Work out the finished part from the listing and answer in its coordinate system (mm). Round coordinates to 2 decimals unless told otherwise and drop trailing zeros. Write each loop counter-clockwise with the first axis right and the second up, starting at its lowest first coordinate (ties: lowest second). Pieces come first, ordered by that corner, then holes. Notation, with made-up numbers: (46.5, 1.25) - (52.5, 1.25) arc R27 ccw to (52.5, 28.25) - close; hole circle Ø1 at (17, -40). An arc over 180 degrees is marked (long way). Write item = value, one per line. Start each with the question number.
from build123d import *

# Parameters (mm, degrees)
SKETCH2_R                    = 12.7
BOSS_EXTRUDE1_DEPTH          = 0.79375
SKETCH3_R                    = 9.525
CUT_EXTRUDE1_DEPTH           = 1.79375
SKETCH4_W                    = 22.318168974
SKETCH4_H                    = 8.357131245
CUT_REVOLVE1_ANGLE           = 45
CUT_REVOLVE1_OTHER_WAY_ANGLE = 45


with BuildPart() as part:
    # Sketch2 → Boss-Extrude1 (new body)
    with BuildSketch(Plane(origin=(0, 0, 0), x_dir=(1, 0, 0), z_dir=(0, 1, 0))):
        Circle(SKETCH2_R)
    extrude(amount=BOSS_EXTRUDE1_DEPTH)

    # Sketch3 → Cut-Extrude1 (cut, through all)
    with BuildSketch(Plane(origin=(0, 0.79375, 0), x_dir=(1, 0, 0), z_dir=(0, 1, 0))):
        Circle(SKETCH3_R)
    extrude(amount=-CUT_EXTRUDE1_DEPTH, mode=Mode.SUBTRACT)

    # Sketch4 → Cut-Revolve1 (revolve, cut)
    with BuildSketch(Plane(origin=(0, 0, 0), x_dir=(0, 0, -1), z_dir=(1, 0, 0))):
        with Locations((-11.159084487, 3.258563731)):
            Rectangle(SKETCH4_W, SKETCH4_H)
    revolve(axis=Axis((0, -0.920001892, 0), (0, 1, 0)), revolution_arc=CUT_REVOLVE1_ANGLE, mode=Mode.SUBTRACT)

    # Sketch4 → Cut-Revolve1 other way (revolve, cut)
    with BuildSketch(Plane(origin=(0, 0, 0), x_dir=(0, 0, -1), z_dir=(1, 0, 0))):
        with Locations((-11.159084487, 3.258563731)):
            Rectangle(SKETCH4_W, SKETCH4_H)
    revolve(axis=Axis((0, -0.920001892, 0), (0, -1, 0)), revolution_arc=CUT_REVOLVE1_OTHER_WAY_ANGLE, mode=Mode.SUBTRACT)


solid = part.part
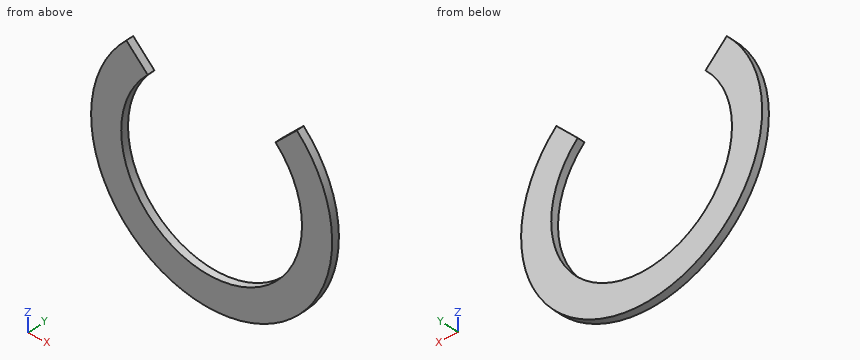
1. Consider line 1 (X direction, y = 0.5, z = 0) (3 decimals); line 2 (Z direction, x = 0, y = 0.55) (3 decimals); line 3 (Z direction, x = 8.5, y = 0.6). Determine where each line is inside the solid, lowest interval first.
2. Find section B-B on x = 7.25. Give the vertices of the cut face in (y, z).
3. Find section A-A on z = 0. Give the vertices of the cut face in (x, y) (3 decimals).
4. Find section C-C on y = 0.15. Give the vertices of the cut face in (x, z) (3 decimals).
5. Find section D-D on x = 0. Give the vertices of the cut face in (y, z) (3 decimals).
Answer key:
q1.line_1 = -12.7 to -9.525, 9.525 to 12.7
q1.line_2 = -12.7 to -9.525
q1.line_3 = -9.44 to -4.3, 4.3 to 8.5
q2.outline = (0, -10.43) - (0.79, -10.43) - (0.79, -6.18) - (0, -6.18) - close; (0, 6.18) - (0.79, 6.18) - (0.79, 7.25) - (0, 7.25) - close
q3.outline = (-12.7, 0) - (-9.525, 0) - (-9.525, 0.794) - (-12.7, 0.794) - close; (9.525, 0) - (12.7, 0) - (12.7, 0.794) - (9.525, 0.794) - close
q4.outline = (-8.98, 8.98) arc R12.7 ccw (long way) to (8.98, 8.98) - (6.735, 6.735) arc R9.525 cw (long way) to (-6.735, 6.735) - close
q5.outline = (0, -12.7) - (0.794, -12.7) - (0.794, -9.525) - (0, -9.525) - close
